from build123d import *

# Parameters (mm, degrees)
F0_W      = 600
F0_H      = 263.0605769157
F1_DEPTH  = 50
F2_SIZE   = 50
F3_SIZE   = 50
F4_R      = 25
F5_DEPTH  = 250
F6_R      = 7.5
F7_DEPTH  = 50
F8_W      = 15
F8_H      = 60
F9_DEPTH  = 250
F10_R     = 25
F10_R_2   = 7.5
F11_DEPTH = 20


# Not quite as in the source:
# - a fillet or chamfer that OpenCascade refuses, or shapes differently, is made with other operations: its cross-section is extruded or revolved along the edge and cut away or added


with BuildPart() as f1:
    # F0 (on Front) → F1 (new body)
    with BuildSketch(Plane.XZ):
        Polygon((505.5267233402, 46.2662550807), (-494.4732766598, 46.2662550807), (-494.4732766598, -83.7337449193), (-344.4732766598, -83.7337449193), (-344.4732766598, -453.7337449193), (-294.4732766598, -453.7337449193), (-294.4732766598, -396.794321835), (305.5267233402, -396.794321835), (305.5267233402, -453.7337449193), (355.5267233402, -453.7337449193), (355.5267233402, -83.7337449193), (505.5267233402, -83.7337449193), align=None)
        with Locations((5.5267233402, -215.2640333772)):
            Rectangle(F0_W, F0_H, mode=Mode.SUBTRACT)
    extrude(amount=F1_DEPTH)

    # F2
    f2_edges = [f1.edges().sort_by_distance(p)[0] for p in [
        (505.526723, -25, -83.733745),
    ]]
    chamfer(f2_edges, length=F2_SIZE)

    # F3
    f3_edges = [f1.edges().sort_by_distance(p)[0] for p in [
        (-494.473277, -25, -83.733745),
    ]]
    chamfer(f3_edges, length=F3_SIZE)

    # F4 (on face) → F5 (join)
    with BuildSketch(Plane.XZ.offset(50)):
        with BuildLine():
            ThreePointArc((-467.4732766598, 46.2662550807), (-485.1509461895, 3.588585551), (-442.4732766598, 21.2662550807))
            ThreePointArc((-442.4732766598, 21.2662550807), (-449.7956071302, 38.9439246104), (-467.4732766598, 46.2662550807))
        make_face()
        with Locations((-415.4736002376, 21.0828103085)):
            Circle(F4_R)
        with Locations((-363.4739238154, 20.8993655363)):
            Circle(F4_R)
        with Locations((-311.4742473932, 20.7159207642)):
            Circle(F4_R)
        with Locations((-259.474570971, 20.532475992)):
            Circle(F4_R)
        with Locations((-207.4748945487, 20.3490312198)):
            Circle(F4_R)
        with Locations((-155.4752181265, 20.1655864476)):
            Circle(F4_R)
        with Locations((-103.4755417043, 19.9821416755)):
            Circle(F4_R)
        with Locations((-51.4758652821, 19.7986969033)):
            Circle(F4_R)
        with Locations((0.5238111401, 19.6152521311)):
            Circle(F4_R)
        with Locations((52.5234875624, 19.4318073589)):
            Circle(F4_R)
        with Locations((104.5231639846, 19.2483625868)):
            Circle(F4_R)
        with Locations((156.5228404068, 19.0649178146)):
            Circle(F4_R)
        with Locations((208.522516829, 18.8814730424)):
            Circle(F4_R)
        with Locations((260.5221932512, 18.6980282702)):
            Circle(F4_R)
        with Locations((312.5218696735, 18.5145834981)):
            Circle(F4_R)
        with Locations((364.5215460957, 18.3311387259)):
            Circle(F4_R)
        with Locations((416.5212225179, 18.1476939537)):
            Circle(F4_R)
        with Locations((468.5208989401, 17.9642491815)):
            Circle(F4_R)
    extrude(amount=F5_DEPTH)

    # F6 (on face) → F7 (join)
    with BuildSketch(Plane(origin=(0, 0, -453.7337449193), x_dir=(1, 0, 0), z_dir=(0, 0, -1))):
        with Locations((-320.3388154507, 25)):
            Circle(F6_R)
        with Locations((330.5267233402, 25)):
            Circle(F6_R)
    extrude(amount=F7_DEPTH)

    # F8 (on face) → F9 (join)
    with BuildSketch(Plane.XZ.offset(50)):
        with Locations((-321.9732766598, -233.7337449193)):
            Rectangle(F8_W, F8_H)
        with Locations((321.9732766598, -233.7337449193)):
            Rectangle(F8_W, F8_H)
    extrude(amount=F9_DEPTH)

    # F10 (on face) → F11 (join)
    with BuildSketch(Plane(origin=(0, 0, -503.7337449193), x_dir=(1, 0, 0), z_dir=(0, 0, -1))):
        with Locations((-320.3388154507, 25)):
            Circle(F10_R)
        with Locations((-320.3388154507, 25)):
            Circle(F10_R_2, mode=Mode.SUBTRACT)
        with Locations((-320.3388154507, 25)):
            Circle(F10_R_2)
        with Locations((330.5267233402, 25)):
            Circle(F10_R)
    extrude(amount=F11_DEPTH)

    # F12: fillet of radius 20 on 2 edges, made by hand

    # F12_s1 → F12_t2 (revolve, cut)
    with BuildSketch(Plane.XZ.offset(25)):
        with BuildLine():
            ThreePointArc((-295.3388154507, -523.5768797523), (-300.3388154507, -510.348123197), (-312.8388154507, -503.7337449193))
            Line((-312.8388154507, -503.7337449193), (-295.3388154507, -503.7337449193))
            Line((-295.3388154507, -503.7337449193), (-295.3388154507, -523.5768797523))
        make_face()
    revolve(axis=Axis((-320.3388154507, -25, -503.7337449193), (0, 0, -1)), mode=Mode.SUBTRACT)

    # F12_s3 → F12_t4 (revolve, cut)
    with BuildSketch(Plane.XZ.offset(25)):
        with BuildLine():
            ThreePointArc((338.0267233402, -503.7337449193), (350.5267233402, -510.348123197), (355.5267233402, -523.5768797523))
            Line((355.5267233402, -523.5768797523), (355.5267233402, -503.7337449193))
            Line((355.5267233402, -503.7337449193), (338.0267233402, -503.7337449193))
        make_face()
    revolve(axis=Axis((330.5267233402, -25, -503.7337449193), (0, 0, -1)), mode=Mode.SUBTRACT)

    # F13: F1 across face


with BuildPart() as f1_1:
    add(f1.part)
    add(f1.part.mirror(Plane(origin=(104.5231639846, -300, 19.2483625868), x_dir=(1, 0, 0), z_dir=(0, -1, 0))))


solid = f1_1.part
Could you check a few things on this model? Use its own coordinates, in mm. A direction names the side the tool comes from. Give positions to 0.01 mm unless a question says otherwise; leave off trailing zeros. Order: outer loops, then holes, each group sorted by start corner. A loop starts at its lowest first (then second) coordinate and runs counter-clockwise, first axis right, second up.
1. Suppose I cut it at D-D (x = 8). List the corners of the cut face in (y, z) for me, plus the area to 3 significant figures.
2. Suppose I cut it at A-A (z = -328). List the corners of the cut face in (x, y) for me, plus the area to 3 significant figures.
3. Suppose I cut it at C-C (y = -154). Give the number of separate pieces and of enclosed holes in the cut face, plus the area to 3 significant figures.
4. We'd pull the mould along X, two halves only. Please class faces 5 (the flat face through (-494.473, -25, 7)), 6 (the flat face through (-294.473, -25, -217)), 7 (the flat face through (355.527, -25, -271)), 8 (the flat face through (1, -25, -346.794)): pulls with the +X half, pulls with the -X half, needs draft (parallel to the pull), parting line crosses it, or undercut.
5. For faces 1 (the flat face through (-344.473, -575, -266)), 2 (the flat face through (1, -575, -396.794)), 3 (the flat face through (1, -575, -346.794)), 4 (the flat face through (-314, -581, -453.734)), which set-ups out of +Z, -Z, +X, -X, +Y, -Y let a thin tool reach every point of the face, with its end or its side?
6. Will these pins go through, and if not, where does the flat tip stop? P1, Ø10, axis at x = -376, y = -336, coming from the +Z side; P2, Ø12, axis at x = -318.5, y = -230.5, coming from the -Z side; P3, Ø25, axis at x = 391, y = -577.5, coming from the -Z side.
7. I need wall thicknesses on L1, parallel to X at y = -30, z = -442.5; L2, parallel to X at y = -407.5, z = -244; L3, parallel to Y at x = 152.5, z = -42. Which ranges of each line are inside material? Lowest first, please.
8. Suppose I cut it at B-B (x = 153). List the corners of the cut face in (y, z) for me, plus the area to 3 significant figures.
Solved:
1. outline: (-600, -396.79) - (-550, -396.79) - (-550, -346.79) - (-600, -346.79) - close; (-600, -83.73) - (-550, -83.73) - (-550, -4.24) - (-50, -4.24) - (-50, -83.73) - (0, -83.73) - (0, 46.27) - (-50, 46.27) - (-50, 43.47) - (-550, 43.47) - (-550, 46.27) - (-600, 46.27) - close; (-50, -396.79) - (0, -396.79) - (0, -346.79) - (-50, -346.79) - close
1. area: 41,900 mm2
2. outline: (-344.47, -600) - (-294.47, -600) - (-294.47, -550) - (-344.47, -550) - close; (-344.47, -50) - (-294.47, -50) - (-294.47, 0) - (-344.47, 0) - close; (305.53, -600) - (355.53, -600) - (355.53, -550) - (305.53, -550) - close; (305.53, -50) - (355.53, -50) - (355.53, 0) - (305.53, 0) - close
2. area: 10,000 mm2
3. separate pieces: 21
3. enclosed holes: 0
3. area: 39,100 mm2
4. face 5: pulls with the -X half
4. face 6: undercut
4. face 7: pulls with the +X half
4. face 8: undercut
5. face 1: -X, +Y, -Y
5. face 2: -Z, +Y, -Y
5. face 3: +Y, -Y
5. face 4: none
6. P1: stops at z = 44.74
6. P2: stops at z = -263.73
6. P3: stops at z = -83.73
7. L1: x = -344.47 to -294.47, 305.53 to 355.53
7. L2: x = -329.47 to -314.47, 314.47 to 329.47
7. L3: y = -600 to -550, -50 to 0
8. outline: (-600, -396.79) - (-550, -396.79) - (-550, -346.79) - (-600, -346.79) - close; (-600, -83.73) - (-550, -83.73) - (-550, -5.69) - (-50, -5.69) - (-50, -83.73) - (0, -83.73) - (0, 46.27) - (-50, 46.27) - (-50, 43.82) - (-550, 43.82) - (-550, 46.27) - (-600, 46.27) - close; (-50, -396.79) - (0, -396.79) - (0, -346.79) - (-50, -346.79) - close
8. area: 42,800 mm2
